The listing builds one solid part. Answer for the finished solid, in the listing's coordinates (mm). Give positions to 0.01 mm unless a question says otherwise; leave off trailing zeros. Write each loop counter-clockwise with the first axis right and the second up, starting at its lowest first coordinate (ties: lowest second). Pieces come first, ordered by that corner, then holes. Notation, with made-up numbers: (66.25, 72.5) -> (118.25, 72.5) arc R16 ccw to (118.25, 76.5) -> close; hole circle Ø7 at (31, 12). An arc over 180 degrees is marked (long way). One line per question, with ' | ' between items.
from build123d import *

# Parameters (mm, degrees)
SKETCH1_R          = 57.15
EXTRUDE1_DEPTH     = 17.526
SKETCH2_R          = 4.2164
CUT_EXTRUDE2_DEPTH = 17.526
CIRPATTERN1_COUNT  = 8


with BuildPart() as part:
    # Sketch1 → Extrude1 (new body)
    with BuildSketch(Plane(origin=(0, 0, 0), x_dir=(1, 0, 0), z_dir=(0, 1, 0))):
        with Locations(Location((0, 0, 0), (0, 0, 270))):
            Circle(SKETCH1_R)
    extrude(amount=EXTRUDE1_DEPTH)

    # Sketch2 → Cut-Extrude2 (cut)
    with BuildSketch(Plane(origin=(0, 0, 0), x_dir=(1, 0, 0), z_dir=(0, 1, 0))):
        with Locations(Location((0, 46.101, 0), (0, 0, 270))):
            Circle(SKETCH2_R)
    cut_extrude2 = extrude(amount=CUT_EXTRUDE2_DEPTH, mode=Mode.SUBTRACT)

    # CirPattern1: Cut-Extrude2 ×8 about axis
    cirpattern1_axis = Axis((0, 0, 0), (0, 1, 0))
    for i in range(1, CIRPATTERN1_COUNT):
        add(cut_extrude2.rotate(cirpattern1_axis, i * 360 / CIRPATTERN1_COUNT), mode=Mode.SUBTRACT)


solid = part.part
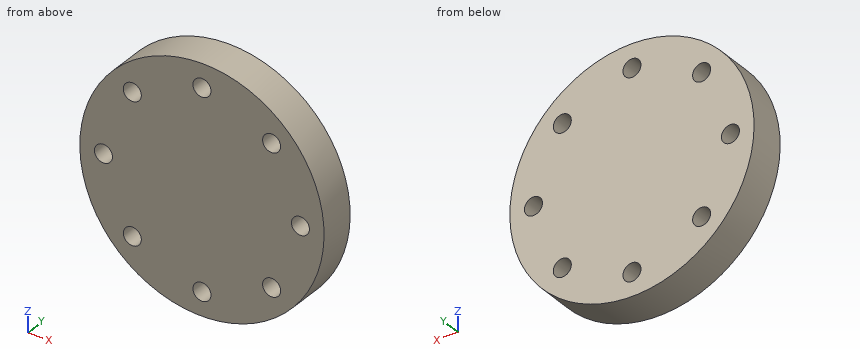
Item 1: Find section B-B (x = 0). Write down the section's boundary in (y, z).
Answers below:
outline: (0, -57.15) -> (17.53, -57.15) -> (17.53, -50.32) -> (0, -50.32) -> close; (0, -41.88) -> (17.53, -41.88) -> (17.53, 41.88) -> (0, 41.88) -> close; (0, 50.32) -> (17.53, 50.32) -> (17.53, 57.15) -> (0, 57.15) -> close
Item 2: Flat-ended cylindrical pins translate along their axes: pin 1 (6 mm diameter, centred on y = 3, z = -33, fed in from -X); pin 2 (11 mm diameter, centred on x = -32.6, z = -32.6, fed in from -Y); pin 3 (4 mm diameter, centred on x = -13.5, y = 9, fed in from -Z); pin 4 (1.5 mm diameter, centred on y = 15.5, z = 24.5, fed in from +X). Find the tip coordinate at first contact, or state that the pin passes through.
Answers below:
pin 1: x = -48.64 | pin 2: y = 0 | pin 3: z = -55.98 | pin 4: x = 51.98
Item 3: Find section A-A (z = 0). Write down the section's boundary in (x, y), then the cut area to 3 significant figures.
Answers below:
outline: (-57.15, 0) -> (-50.32, 0) -> (-50.32, 17.53) -> (-57.15, 17.53) -> close; (-41.88, 0) -> (41.88, 0) -> (41.88, 17.53) -> (-41.88, 17.53) -> close; (50.32, 0) -> (57.15, 0) -> (57.15, 17.53) -> (50.32, 17.53) -> close | area: 1,710 mm²
Item 4: Find section D-D (y = 4.75). Count the separate pieces of the cut face and the enclosed holes in it, then the cut area to 3 significant figures.
Answers below:
separate pieces: 1 | enclosed holes: 8 | area: 9,810 mm²
Item 5: Find section C-C (z = 49). Write down the section's boundary in (x, y).
Answers below:
outline: (-29.41, 0) -> (-3.06, 0) -> (-3.06, 17.53) -> (-29.41, 17.53) -> close; (3.06, 0) -> (29.41, 0) -> (29.41, 17.53) -> (3.06, 17.53) -> close
Item 6: Consider line 1 (Z direction, x = 33, y = 8); line 2 (Z direction, x = -36, y = 2); line 3 (X direction, y = 16.25, z = 2) (3 decimals). Determine where each line is inside the solid, lowest interval first. Write a range as [from, to].
Answers below:
line 1: [-46.66, -36.8], [-28.4, 28.4], [36.8, 46.66] | line 2: [-44.39, -35.09], [-30.11, 30.11], [35.09, 44.39] | line 3: [-57.115, -49.813], [-42.389, 42.389], [49.813, 57.115]
